Can you work these out from the model? Positions are in its coordinate system, mm. Give positions to 0.01 mm unless a question says otherwise; leave off trailing zeros. Order: outer loops, then holes, each group sorted by start corner. A loop starts at its lowest first (then second) coordinate and runs counter-clockwise, first axis right, second up. Notation, with made-up numbers: M 18,52 L 31,52 A12 ccw 31,66 Z; hole C 12.25,-38 d10. An arc over 180 degrees is marked long. Answer as a JSON object with one key per item and string values.
```python
from build123d import *

# Parameters (mm, degrees)
BOSS_EXTRUDE1_DEPTH = 5.588
FILLET1_R           = 5.08
FILLET3_R           = 7.62
SKETCH3_R           = 2.5273
SKETCH3_W           = 5.588
SKETCH3_H           = 12.7
CUT_EXTRUDE2_DEPTH  = 138.960432195
BOSS_EXTRUDE3_DEPTH = 5.588


with BuildPart() as part:
    # Sketch1 → Boss-Extrude1 (new body)
    with BuildSketch(Plane.XY):
        with BuildLine():
            Line((-108.048552, 85.600032), (-30.737556, 85.600032))
            Line((-30.737556, 85.600032), (-30.737556, 67.394105789))
            add(Edge.make_bspline(
                [(-30.737556, 67.394105789), (-19.663465212, 56.532474897), (0, 56.532474897)],
                knots=[0, 0, 0, 1, 1, 1], degree=2))
            add(Edge.make_bspline(
                [(30.737556, 67.394105789), (19.663465212, 56.532474897), (0, 56.532474897)],
                knots=[0, 0, 0, 1, 1, 1], degree=2))
            Line((30.737556, 67.394105789), (30.737556, 85.600032))
            Line((30.737556, 85.600032), (108.048552, 85.600032))
            Line((108.048552, 85.600032), (108.048552, 0))
            Line((108.048552, 0), (-108.048552, 0))
            Line((-108.048552, 0), (-108.048552, 85.600032))
        make_face()
    extrude(amount=BOSS_EXTRUDE1_DEPTH)

    # Fillet1
    fillet1_edges = [part.edges().sort_by_distance(p)[0] for p in [
        (30.737556, 85.600032, 2.794),
        (108.048552, 85.600032, 2.794),
        (108.048552, 0, 2.794),
        (-108.048552, 0, 2.794),
        (-108.048552, 85.600032, 2.794),
        (-30.737556, 85.600032, 2.794),
    ]]
    fillet(fillet1_edges, radius=FILLET1_R)

    # Fillet3
    fillet3_edges = [part.edges().sort_by_distance(p)[0] for p in [
        (30.737556, 67.394105789, 2.794),
        (-30.737556, 67.394105789, 2.794),
    ]]
    fillet(fillet3_edges, radius=FILLET3_R)

    # Sketch3 → Cut-Extrude2 (cut, through all)
    with BuildSketch(Plane.XY):
        with Locations((-99.031552, 25.4)):
            Circle(SKETCH3_R)
        with Locations((99.031552, 25.4)):
            Circle(SKETCH3_R)
        with Locations((-99.031552, 14.208252)):
            Rectangle(SKETCH3_W, SKETCH3_H)
        with Locations((99.031552, 14.208252)):
            Rectangle(SKETCH3_W, SKETCH3_H)
        with Locations((-99.031552, 36.591748)):
            Rectangle(SKETCH3_W, SKETCH3_H)
        with Locations((99.031552, 36.591748)):
            Rectangle(SKETCH3_W, SKETCH3_H)
    extrude(amount=CUT_EXTRUDE2_DEPTH, mode=Mode.SUBTRACT)

    # Sketch5 → Boss-Extrude3 (add)
    with BuildSketch(Plane.XY.offset(5.588)):
        with BuildLine():
            ThreePointArc((-102.968552, 0), (-106.560654448, 1.487897552), (-108.048552, 5.08))
            Line((-108.048552, 5.08), (-108.048552, -3.683))
            ThreePointArc((-108.048552, -3.683), (-106.560654448, -7.275102448), (-102.968552, -8.763))
            Line((-102.968552, -8.763), (102.968552, -8.763))
            ThreePointArc((102.968552, -8.763), (106.560654448, -7.275102448), (108.048552, -3.683))
            Line((108.048552, -3.683), (108.048552, 5.08))
            ThreePointArc((108.048552, 5.08), (106.560654448, 1.487897552), (102.968552, 0))
            Line((102.968552, 0), (28.41625, 0))
            Line((28.41625, 0), (28.41625, -5.842))
            Line((28.41625, -5.842), (5.55625, -5.842))
            Line((5.55625, -5.842), (5.55625, 0))
            Line((5.55625, 0), (-5.55625, 0))
            Line((-5.55625, 0), (-5.55625, -5.842))
            Line((-5.55625, -5.842), (-28.41625, -5.842))
            Line((-28.41625, -5.842), (-28.41625, 0))
            Line((-28.41625, 0), (-102.968552, 0))
        make_face()
    extrude(amount=-BOSS_EXTRUDE3_DEPTH)


solid = part.part
```
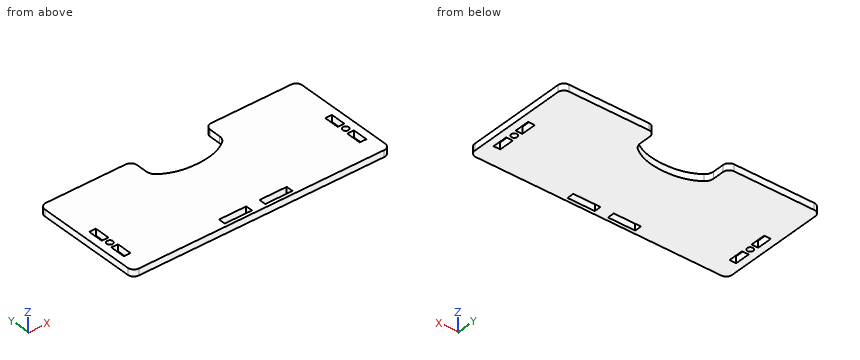
1) I need wall thicknesses on L1, parallel to X at y = 25.4, z = 2.3; L2, parallel to X at y = 42.5, z = 2.45; L3, parallel to Y at x = 19.5, z = 5.3. Which ranges of each line are inside material? Lowest first, please.
Results found:
{"L1": "x = -108.05 to -101.56, -96.5 to 96.5, 101.56 to 108.05", "L2": "x = -108.05 to -101.83, -96.24 to 96.24, 101.83 to 108.05", "L3": "y = -8.76 to -5.84, 0 to 60.01"}
2) I want a section at D-D on y = 25.4. Write out the boundary of the cut face in (x, z).
Results found:
{"outline": "M -108.05,0 L -101.56,0 L -101.56,5.59 L -108.05,5.59 Z; M -96.5,0 L 96.5,0 L 96.5,5.59 L -96.5,5.59 Z; M 101.56,0 L 108.05,0 L 108.05,5.59 L 101.56,5.59 Z"}
3) I want a section at A-A on y = 73. Write out the boundary of the cut face in (x, z), and give its area (3 significant figures).
Results found:
{"outline": "M -108.05,0 L -30.74,0 L -30.74,5.59 L -108.05,5.59 Z; M 30.74,0 L 108.05,0 L 108.05,5.59 L 30.74,5.59 Z", "area": "864 mm²"}
4) I'm going to push a flat-ended pin straight in: pin 1 Ø8 at (x, y) = (-35.5, 46.5) entering from -Z. Where does the tip first touch, or does it pass through?
Results found:
{"pin 1": "stops at z = 0"}
5) I want a section at C-C on z = 4.55. Count the separate pieces of the cut face and the enclosed holes in it, and give its area (3 significant figures).
Results found:
{"separate pieces": "1", "enclosed holes": "8", "area": "18,200 mm²"}
6) I want a section at B-B on y = 40.5. Write out the boundary of the cut face in (x, z), and give its area (3 significant figures).
Results found:
{"outline": "M -108.05,0 L -101.83,0 L -101.83,5.59 L -108.05,5.59 Z; M -96.24,0 L 96.24,0 L 96.24,5.59 L -96.24,5.59 Z; M 101.83,0 L 108.05,0 L 108.05,5.59 L 101.83,5.59 Z", "area": "1,150 mm²"}
